For this review, take the finished solid that the model builds, in its own axes (mm). Coordinates: 2 decimals unless noted, no trailing zeros. Order: outer loops, then holes, each group sorted by start corner. A loop starts at its lowest first (then second) coordinate and runs counter-clockwise, first axis right, second up. Notation, with made-up numbers: (26.5, 86) -> (57.5, 86) arc R25 cw to (57.5, 102) -> close; hole circle Ø1 at (64.5, 57). An arc over 180 degrees is marked (long way). Write item = value, one per line. Start each with the question number.
1) Consider section A-A on y = 63. Give the boundary of the cut face in (x, z).
2) Insertion check: pin 1 Ø0.9 at (x, z) = (52.5, 1) entering from -Y; pin 2 Ø1.2 at (x, y) = (93.25, 5) entering from -Z; pin 3 Ø1.5 at (x, z) = (84, 1.5) entering from -Y; pin 4 Ø0.9 at (y, z) = (9.5, 2) entering from +X. Each pin has a flat end and moves straight along its axis. Give the tip position at first contact, or say it passes through.
3) Consider section C-C on x = 15. Give the boundary of the cut face in (y, z).
4) Wall thickness on probe 1 along Y at (x, z) = (8, 2.2); probe 2 along Y at (x, z) = (53, 1); probe 3 along X at (y, z) = (5, 1.55): over which ranges is each line inside the solid? List them lowest first. Write a range as [from, to].
5) Consider section D-D on z = 2.4. State how many separate pieces and enclosed holes the cut face has, and give its area (3 significant figures).
6) Consider section B-B on y = 16.5. Give the boundary of the cut face in (x, z), and give its area (4 significant figures).
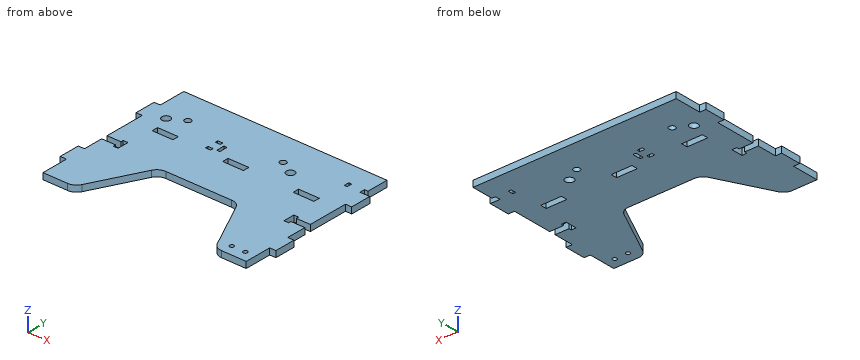
Autodesk Inventor part; units mm, degrees
ref_plane "YZ Plane" through (0, 0, 0) normal (1, 0, 0) x (0, 1, 0)
ref_plane "XZ Plane" through (0, 0, 0) normal (0, 1, 0) x (-1, 0, 0)
ref_plane "XY Plane" through (0, 0, 0) normal (0, 0, 1) x (1, 0, 0)
sketch "Sketch1" plane through (0, 0, 0) normal (0, 0, 1) x (1, 0, 0)
  line L0 (0, 0) -> (98, 0)
  line L1 (98, 0) -> (98, 78)
  line L2 (98, 78) -> (0, 78)
  line L3 (0, 78) -> (0, 0)
  line L4 (-3, 65) -> (101, 65)
  line L5 (101, 65) -> (101, 55)
  line L6 (101, 55) -> (-3, 55)
  line L7 (-3, 55) -> (-3, 65)
  line L8 (101, 23) -> (101, 13)
  line L9 (-3, 13) -> (-3, 23)
  line L10 (68, 30) -> (30, 30)
  line L11 (15, 0) -> (30, 30)
  line L12 (83, 0) -> (68, 30)
  line L13 (15, 0) -> (83, 0)
  line L14 (-3, 23) -> (0, 23)
  line L15 (98, 23) -> (101, 23)
  line L16 (101, 13) -> (98, 13)
  line L17 (0, 13) -> (-3, 13)
  dimension "d0" = 98
  dimension "d1" = 78
  dimension "d171" = 104
  dimension "d172" = 3
  dimension "d173" = 10
  dimension "d174" = 13
  dimension "d175" = 10
  dimension "d177" = 3
  dimension "d181" = 30
  dimension "d182" = 30
  dimension "d183" = 30
  dimension "d184" = 15
  dimension "d185" = 15
  dimension "d186" = 10
  dimension "d187" = 13
  dimension "d188" = 13
extrude "Extrusion1" add sketch "Sketch1" along normal blind 3 contours L3 L6 L1 L0 L12 L10 L11 | L17 L9 L14 L3 | L6 L7 L4 L3 | L3 L4 L1 L6 | L1 L15 L8 L16 | L3 L2 L1 L4 | L1 L4 L5 L6
fillet "圓角4" radius 5 4 edges at (15, 0, 1.5) (30, 30, 1.5) (68, 30, 1.5) (83, 0, 1.5)
sketch "草圖13" plane through (0, 0, 3) normal (0, 0, 1) x (1, 0, 0)
  line L0 (98, 55) -> (98, 23)
  line L1 (0, 78) -> (98, 78)
  line L2 (0, 65) -> (0, 78)
  line L3 (0, 23) -> (0, 55)
  line L4 (10, 52) -> (20, 52)
  line L5 (20, 52) -> (20, 49)
  line L6 (20, 49) -> (10, 49)
  line L7 (10, 49) -> (10, 52)
  line L8 (44, 52) -> (54, 52)
  line L9 (54, 52) -> (54, 49)
  line L10 (54, 49) -> (44, 49)
  line L11 (44, 49) -> (44, 52)
  line L12 (78, 52) -> (88, 52)
  line L13 (88, 52) -> (88, 49)
  line L14 (88, 49) -> (78, 49)
  line L15 (78, 49) -> (78, 52)
  dimension "d190" = 10
  dimension "d191" = 10
  dimension "d192" = 3
  dimension "d193" = 26
  dimension "d194" = 10
  dimension "d195" = 10
  dimension "d196" = 10
  dimension "d198" = 44
extrude "擠出6" cut sketch "草圖13" against normal through all
sketch "草圖14" plane through (0, 0, 3) normal (0, 0, 1) x (1, 0, 0)
  line L0 (0, 78) -> (98, 78)
  line L1 (0, 65) -> (0, 78)
  point P0 (8, 59)
  point P1 (68, 59)
  dimension "d201" = 8
  dimension "d202" = 19
  dimension "d203" = 60
hole "孔5" at (8, 59, 3) at (68, 59, 3) direction (0, 0, -1) diameter 4 end through all
sketch "草圖15" plane through (0, 0, 3) normal (0, 0, 1) x (1, 0, 0)
  line L0 (0, 78) -> (98, 78)
  line L1 (0, 65) -> (0, 78)
  point P0 (15, 63)
  point P1 (61, 63)
  dimension "d211" = 15
  dimension "d212" = 15
  dimension "d213" = 46
hole "孔6" at (15, 63, 3) at (61, 63, 3) direction (0, 0, -1) diameter 3 end through all
sketch "草圖16" plane through (0, 0, 3) normal (0, 0, 1) x (1, 0, 0)
  line L0 (98, 0) -> (86.0902, 0)
  line L1 (98, 13) -> (98, 0)
  point P0 (93.25, 5)
  point P1 (86.75, 5)
  dimension "d221" = 5
  dimension "d222" = 4.75
  dimension "d223" = 6.5
hole "孔7" at (93.25, 5, 3) at (86.75, 5, 3) direction (0, 0, -1) diameter 2 end through all
sketch "草圖17" plane through (0, 0, 3) normal (0, 0, 1) x (1, 0, 0)
  line L0 (98, 55) -> (98, 23)
  line L1 (0, 23) -> (0, 55)
  line L2 (11.9098, 0) -> (0, 0)
  line L3 (0, 35.5) -> (9, 35.5)
  line L4 (9, 35.5) -> (9, 32.5)
  line L5 (9, 32.5) -> (0, 32.5)
  line L6 (0, 32.5) -> (0, 35.5)
  line L7 (9, 36.75) -> (6.7, 36.75)
  line L8 (6.7, 36.75) -> (6.7, 31.25)
  line L9 (6.7, 31.25) -> (9, 31.25)
  line L10 (9, 31.25) -> (9, 36.75)
  line L11 (89, 35.5) -> (98, 35.5)
  line L12 (98, 35.5) -> (98, 32.5)
  line L13 (98, 32.5) -> (89, 32.5)
  line L14 (89, 32.5) -> (89, 35.5)
  line L15 (89, 36.75) -> (91.3, 36.75)
  line L16 (91.3, 36.75) -> (91.3, 31.25)
  line L17 (91.3, 31.25) -> (89, 31.25)
  line L18 (89, 31.25) -> (89, 36.75)
  dimension "d231" = 9
  dimension "d233" = 3
  dimension "d234" = 32.5
  dimension "d235" = 2.3
  dimension "d236" = 5.5
  dimension "d237" = 1.25
  dimension "d239" = 9
  dimension "d240" = 2.3
extrude "擠出7" cut sketch "草圖17" against normal through all
sketch "草圖18" plane through (0, 0, 3) normal (0, 0, 1) x (1, 0, 0)
  line L0 (0, 35.5) -> (0, 55)
  line L1 (10, 52) -> (20, 52)
  line L2 (37, 57.75) -> (38.5, 57.75)
  line L3 (38.5, 57.75) -> (38.5, 53.75)
  line L4 (38.5, 53.75) -> (37, 53.75)
  line L5 (37, 53.75) -> (37, 57.75)
  line L6 (35.25, 57.75) -> (32.75, 57.75)
  line L7 (32.75, 57.75) -> (32.75, 59.15)
  line L8 (32.75, 59.15) -> (35.25, 59.15)
  line L9 (35.25, 59.15) -> (35.25, 57.75)
  line L10 (35.25, 53.75) -> (32.75, 53.75)
  line L11 (32.75, 53.75) -> (32.75, 52.35)
  line L12 (32.75, 52.35) -> (35.25, 52.35)
  line L13 (35.25, 52.35) -> (35.25, 53.75)
  line L14 (98, 65) -> (96.3, 65)
  line L15 (96.3, 65) -> (96.3, 67.5)
  line L16 (96.3, 67.5) -> (98, 67.5)
  line L17 (98, 67.5) -> (98, 65)
  line L18 (90.125, 67.5) -> (88.725, 67.5)
  line L19 (88.725, 67.5) -> (88.725, 65)
  line L20 (88.725, 65) -> (90.125, 65)
  line L21 (90.125, 65) -> (90.125, 67.5)
  dimension "d243" = 37
  dimension "d244" = 1.75
  dimension "d245" = 4
  dimension "d246" = 1.5
  dimension "d247" = 2.5
  dimension "d248" = 1.4
  dimension "d249" = 1.75
  dimension "d250" = 1.4
  dimension "d254" = 1.7
  dimension "d255" = 2.5
  dimension "d256" = 1.4
  dimension "d257" = 6.175
extrude "擠出8" cut sketch "草圖18" against normal through all
properties part number "plastic_part_1"
Answer sheet:
q1.outline = (-3, 0) -> (13.5, 0) -> (13.5, 3) -> (-3, 3) -> close; (16.5, 0) -> (59.5, 0) -> (59.5, 3) -> (16.5, 3) -> close; (62.5, 0) -> (101, 0) -> (101, 3) -> (62.5, 3) -> close
q2.pin_1 = 30
q2.pin_2 = through
q2.pin_3 = 0.18
q2.pin_4 = 98
q3.outline = (1.07, 0) -> (49, 0) -> (49, 3) -> (1.07, 3) -> close; (52, 0) -> (61.5, 0) -> (61.5, 3) -> (52, 3) -> close; (64.5, 0) -> (78, 0) -> (78, 3) -> (64.5, 3) -> close
q4.probe_1 = [0, 31.25], [36.75, 57], [61, 78]
q4.probe_2 = [30, 49], [52, 78]
q4.probe_3 = [0, 17.5], [80.5, 85.75], [87.75, 92.25], [94.25, 98]
q5.separate_pieces = 1
q5.enclosed_holes = 13
q5.area = 5,950 mm2
q6.outline = (-3, 0) -> (23.25, 0) -> (23.25, 3) -> (-3, 3) -> close; (74.75, 0) -> (101, 0) -> (101, 3) -> (74.75, 3) -> close
q6.area = 157.5 mm2
